Input: part model. Units: mm. Frame: model coordinates. Round coordinates to 2 decimals unless told otherwise and drop trailing zeros. Loops run counter-clockwise (first coordinate to the right, second up) from the corner with the lowest first, then second, coordinate; pieces in that order, holes last.
1) Section C-C, the plane x = 8.5. Return loops of the section in (y, z), and give its area (3 significant figures).
2) Ray query, line 1 along Z through (x, y) = (11.5, 0.4); line 2 along X through (y, z) = (0.15, -8); line 3 along Z through (x, y) = (11, 0.35). Return the intervals inside material, ascending.
3) Section B-B, the plane z = 13. Return loops of the section in (x, y).
4) Section A-A, the plane y = 0.25. Return loops of the section in (x, z), and give its area (3 significant figures).
Autodesk Inventor part; units mm, degrees
ref_plane "YZ Plane" through (0, 0, 0) normal (1, 0, 0) x (0, 1, 0)
ref_plane "XZ Plane" through (0, 0, 0) normal (0, 1, 0) x (-1, 0, 0)
ref_plane "XY Plane" through (0, 0, 0) normal (0, 0, 1) x (1, 0, 0)
sketch "スケッチ1" plane through (0, 0, 0) normal (0, 1, 0) x (-1, 0, 0)
  line L0 (-13.5, -15.8718) -> (-13.5, 16.1282)
  circle A0 centre (-11.5, 16.1282) radius 0.8
  line L1 (-13.5, -10.6768) -> (-13.5, 15.3232)
  line L2 (-13.5, 16.1282) -> (-13.5, 10.2382)
  line L3 (-13.5, 10.2382) -> (-13.5, -3.9818)
  line L4 (-13.5, -3.9818) -> (-13.5, -15.8718)
  line L5 (-13.5, -15.8718) -> (-9.5, -15.8718)
  line L6 (-9.5, -15.8718) -> (-9.5, -9.8718)
  circle A1 centre (-11.5, 16.1282) radius 0.8
  line L7 (-18.5, 22.1282) -> (0, 22.1282)
  line L8 (-13.5, -15.8718) -> (-9.5, -15.8718)
  line L9 (-9.5, -15.8718) -> (-9.5, -9.8718)
  line L10 (-9.5, -6.6718) -> (0, -6.6718)
  line L11 (-9.5, -15.8718) -> (-9.5, -6.6718)
  line L12 (0, 22.1282) -> (0, -6.6718)
  line L13 (13.5, -15.8718) -> (13.5, 16.1282)
  line L14 (13.5, -15.8718) -> (9.5, -15.8718)
  line L15 (18.5, 22.1282) -> (0, 22.1282)
  line L16 (9.5, -6.6718) -> (0, -6.6718)
  line L17 (9.5, -15.8718) -> (9.5, -6.6718)
  circle A2 centre (-11.5, -12.8718) radius 1
  circle A3 centre (-11.5, 16.1282) radius 1
  circle A4 centre (11.5, -12.8718) radius 1
  circle A5 centre (-11.5, 16.1282) radius 1
  circle A6 centre (11.5, 16.1282) radius 1
  circle A7 centre (-11.5, -12.8718) radius 1
  circle A8 centre (11.5, -12.8718) radius 1
  circle A9 centre (0, -12.6718) radius 7.5
  spline S0 degree 3 poles (0, -30.8718) (-3.9797, -30.6573) (-6.3943, -30.6605) (-10.2198, -30.5013) (-11.7409, -30.3574) (-14.0031, -29.6154) (-14.9542, -29.1518) (-16.6972, -27.6417) (-17.3717, -26.7721) (-18.3737, -25.0018) (-18.7365, -24.1111) (-19.2696, -22.239) (-19.4316, -21.261) (-19.5, -20.2718) knots 0 0 0 0 1.195654 1.195654 2.243866 2.243866 2.930767 2.930767 3.539935 3.539935 4.077393 4.077393 4.633359 4.633359 4.633359 4.633359
  spline S1 degree 3 poles (19.5, -20.2718) (19.3569, -22.3429) (18.8278, -24.0013) (17.6447, -26.3968) (16.8969, -27.447) (15.0392, -29.0976) (14.097, -29.571) (12.111, -30.2513) (10.9109, -30.4205) (7.3866, -30.667) (4.5667, -30.6246) (0, -30.8718) knots 0 0 0 0 0.622814 0.622814 1.176012 1.176012 1.714262 1.714262 2.395692 2.395692 3.535201 3.535201 3.535201 3.535201
  line L18 (19.5, -10.8718) -> (19.5, -20.2718)
  arc A10 (19.5, -10.8718) -> (18.5, -9.8718) centre (18.5, -10.8718) ccw
  line L19 (13.5, -9.8718) -> (18.5, -9.8718)
  line L20 (13.5, 16.1282) -> (13.5, -9.8718)
  line L21 (18.5, 16.1282) -> (13.5, 16.1282)
  arc A11 (18.5, 16.1282) -> (19.5, 17.1282) centre (18.5, 17.1282) ccw
  line L22 (19.5, 21.1282) -> (19.5, 17.1282)
  arc A12 (19.5, 21.1282) -> (18.5, 22.1282) centre (18.5, 21.1282) ccw
  line L23 (-18.5, 22.1282) -> (18.5, 22.1282)
  arc A13 (-18.5, 22.1282) -> (-19.5, 21.1282) centre (-18.5, 21.1282) ccw
  line L24 (-19.5, 17.1282) -> (-19.5, 21.1282)
  arc A14 (-19.5, 17.1282) -> (-18.5, 16.1282) centre (-18.5, 17.1282) ccw
  line L25 (-13.5, 16.1282) -> (-18.5, 16.1282)
  line L26 (-13.5, -9.8718) -> (-13.5, 16.1282)
  line L27 (-18.5, -9.8718) -> (-13.5, -9.8718)
  arc A15 (-18.5, -9.8718) -> (-19.5, -10.8718) centre (-18.5, -10.8718) ccw
  line L28 (-19.5, -20.2718) -> (-19.5, -10.8718)
  circle A16 centre (-11.5, 16.1282) radius 1
  circle A17 centre (11.5, 16.1282) radius 1
  circle A18 centre (-11.5, -12.8718) radius 1
  circle A19 centre (11.5, -12.8718) radius 1
  circle A20 centre (0, -12.6718) radius 7.5
  spline S2 degree 3 poles (0, -30.8718) (-3.9797, -30.6573) (-6.3943, -30.6605) (-10.2198, -30.5013) (-11.7409, -30.3574) (-14.0031, -29.6154) (-14.9542, -29.1518) (-16.6972, -27.6417) (-17.3717, -26.7721) (-18.3737, -25.0018) (-18.7365, -24.1111) (-19.2696, -22.239) (-19.4316, -21.261) (-19.5, -20.2718) knots 0 0 0 0 1.195654 1.195654 2.243866 2.243866 2.930767 2.930767 3.539935 3.539935 4.077393 4.077393 4.633359 4.633359 4.633359 4.633359
  spline S3 degree 3 poles (19.5, -20.2718) (19.3569, -22.3429) (18.8278, -24.0013) (17.6447, -26.3968) (16.8969, -27.447) (15.0392, -29.0976) (14.097, -29.571) (12.111, -30.2513) (10.9109, -30.4205) (7.3866, -30.667) (4.5667, -30.6246) (0, -30.8718) knots 0 0 0 0 0.622814 0.622814 1.176012 1.176012 1.714262 1.714262 2.395692 2.395692 3.535201 3.535201 3.535201 3.535201
  line L29 (19.5, -10.8718) -> (19.5, -20.2718)
  arc A21 (19.5, -10.8718) -> (18.5, -9.8718) centre (18.5, -10.8718) ccw
  line L30 (13.5, -9.8718) -> (18.5, -9.8718)
  line L31 (13.5, 16.1282) -> (13.5, -9.8718)
  line L32 (18.5, 16.1282) -> (13.5, 16.1282)
  arc A22 (18.5, 16.1282) -> (19.5, 17.1282) centre (18.5, 17.1282) ccw
  line L33 (19.5, 21.1282) -> (19.5, 17.1282)
  arc A23 (19.5, 21.1282) -> (18.5, 22.1282) centre (18.5, 21.1282) ccw
  line L34 (-18.5, 22.1282) -> (18.5, 22.1282)
  arc A24 (-18.5, 22.1282) -> (-19.5, 21.1282) centre (-18.5, 21.1282) ccw
  line L35 (-19.5, 17.1282) -> (-19.5, 21.1282)
  arc A25 (-19.5, 17.1282) -> (-18.5, 16.1282) centre (-18.5, 17.1282) ccw
  line L36 (-13.5, 16.1282) -> (-18.5, 16.1282)
  line L37 (-13.5, -9.8718) -> (-13.5, 16.1282)
  line L38 (-18.5, -9.8718) -> (-13.5, -9.8718)
  arc A26 (-18.5, -9.8718) -> (-19.5, -10.8718) centre (-18.5, -10.8718) ccw
  line L39 (-19.5, -20.2718) -> (-19.5, -10.8718)
  line L40 (1.5, 6.1282) -> (1.5, 0.1282)
  line L41 (-1.5, 6.1282) -> (-1.5, 0.1282)
  line L42 (1.5, 3.1282) -> (-1.5, 3.1282)
  line L43 (13.5, 16.1282) -> (18.5, 16.1282)
  line L44 (-13.5, 16.1282) -> (-18.5, 16.1282)
  line L45 (-18.5, 16.1282) -> (-18.5, 22.1282)
  line L46 (18.5, 16.1282) -> (18.5, 22.1282)
  circle A27 centre (11.5, 16.1282) radius 1
  point P0 (0, 0)
  point P1 (11.5, 16.1282)
  point P2 (0, 3.1282)
  point P3 (4.3, 10.2382)
  point P4 (0, -5.1718)
  point P5 (0, -5.1718)
  point P6 (4.5, -6.6718)
  point P7 (-4.5, -6.6718)
  dimension "d56" = 29
  dimension "d57" = 2
  dimension "d60" = 6
extrude "押し出し1" add sketch "スケッチ1" along normal blind 0.8 contours L0 L25 L45 L7 L12 A9 L10 L11 L6 L5 | A9 L12 L10 | L12 A9 L16 | L12 L15 L46 L21 L13 L14 L17 L16 A9
sketch "スケッチ3" plane through (0, 0.8, 0) normal (0, 1, 0) x (1, 0, 0)
  line L0 (6.4, -15.9282) -> (-6.4, -15.9282)
  line L1 (-6.4, -15.9282) -> (-6.4, -22.1282)
  line L2 (6.4, -22.1282) -> (6.4, -15.9282)
  line L3 (-18.5, -22.1282) -> (18.5, -22.1282)
  point P0 (0, -15.9282)
  point P1 (0, -22.1282)
  dimension "d26" = 12.8
  dimension "d27" = 6.2
extrude "押し出し3" cut sketch "スケッチ3" against normal through all
fillet "フィレット1" radius 2 6 edges at (13.5, 0.4, -15.8718) (-13.5, 0.4, -15.8718) (-18.5, 0.4, 16.1282) (-18.5, 0.4, 22.1282) (18.5, 0.4, 22.1282) (18.5, 0.4, 16.1282)
properties part number "SubBoard"
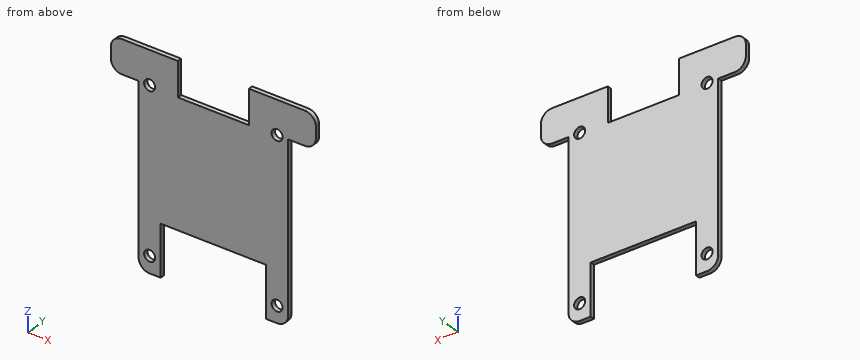
Final values:
1. outline: (0, -6.67) - (0.8, -6.67) - (0.8, 22.13) - (0, 22.13) - close
1. area: 23.0 mm2
2. line 1: z = -15.87 to -13.87, -11.87 to 15.13, 17.13 to 22.13
2. line 2: x = -13.5 to -9.5, 9.5 to 13.5
2. line 3: z = -15.87 to -13.74, -12.01 to 15.26, 16.99 to 22.13
3. outline: (-13.5, 0) - (13.5, 0) - (13.5, 0.8) - (-13.5, 0.8) - close
4. outline: (-18.5, 18.13) arc R2 ccw to (-16.5, 16.13) - (-13.5, 16.13) - (-13.5, -13.87) arc R2 ccw to (-11.5, -15.87) - (-9.5, -15.87) - (-9.5, -6.67) - (9.5, -6.67) - (9.5, -15.87) - (11.5, -15.87) arc R2 ccw to (13.5, -13.87) - (13.5, 16.13) - (16.5, 16.13) arc R2 ccw to (18.5, 18.13) - (18.5, 20.13) arc R2 ccw to (16.5, 22.13) - (6.4, 22.13) - (6.4, 15.93) - (-6.4, 15.93) - (-6.4, 22.13) - (-16.5, 22.13) arc R2 ccw to (-18.5, 20.13) - close; hole circle Ø2 at (-11.5, -12.87); hole circle Ø2 at (-11.5, 16.13); hole circle Ø2 at (11.5, -12.87); hole circle Ø2 at (11.5, 16.13)
4. area: 814 mm2
